```python
from build123d import *

# Parameters (mm, degrees)
F0_W     = 110
F0_H     = 2
F1_DEPTH = 412
F2_W     = 455.0662100537
F2_H     = 4
F3_DEPTH = 16


with BuildPart() as f1:
    # F0 (on Top) → F1 (new body)
    with BuildSketch(Plane.XY):
        with Locations((-49.3745803833, 21.5659940839)):
            Rectangle(F0_W, F0_H)
        Polygon((5.6254196167, 22.5659940839), (5.6254196167, 20.5659940839), (465.6254196127, 100.5659940832), (453.9570552758, 100.5659940832), align=None)
    extrude(amount=F1_DEPTH)

    # F2 (on face) → F3 (join)
    with BuildSketch(Plane(origin=(-3.6453815607, 20.9530753552, 0), x_dir=(-0.9852008911, -0.1714036294, 0), z_dir=(-0.1714036294, 0.9852008911, 0))):
        with Locations((-236.9431667321, 410)):
            Rectangle(F2_W, F2_H)
    extrude(amount=F3_DEPTH)


solid = f1.part
```
Geometry check sheet. Reference: the model listing, model coordinates, mm. A direction names the side the tool comes from. Round coordinates to 2 decimals unless told otherwise and drop trailing zeros. Loops run counter-clockwise (first coordinate to the right, second up) from the corner with the lowest first, then second, coordinate; pieces in that order, holes last. Notation, with made-up numbers: (61.5, 47) - (112.5, 47) arc R9 cw to (112.5, 55) - close; hole circle Ø1 at (16, 6.5). An arc over 180 degrees is marked (long way). Write each question's results on one line, items separated by ' | '. Start each with the question number.
Q1. Gauge pin test, flat ends, axial feed: P1, Ø9.5, axis at x = 457.5, z = 128.5, coming from the +Y side; P2, Ø5, axis at x = 267, z = 229.5, coming from the +Y side; P3, Ø10, axis at x = 342.5, z = 261, coming from the -Y side. Record the tip position at first contact, or that the pin passes through.
Q2. Thickness scan on line 1 (Z direction, x = 53, y = 43); line 2 (Y direction, x = -66.5, z = 181); line 3 (Y direction, x = 182.5, z = 23.5). Record the ranges inside material, lowest first. Write a range as [from, to].
Q3. Cross-section at B-B on x = 13.5. Enter the section's corners in (y, z).
Q4. Access from +Z, -Z, +X, -X, +Y, -Y to the whole of each face (thin tool, end or side, straight path). Record for faces 1 (the flat face through (-50, 20.566, 203)), 2 (the flat face through (232, 70, 408)).
Q5. Cross-section at A-A on z = 117. Enter the section's corners in (x, y).
Answers below:
1) P1: stops at y = 100.57 | P2: stops at y = 68.47 | P3: stops at y = 78.28
2) line 1: z = [408, 412] | line 2: y = [20.57, 22.57] | line 3: y = [51.33, 53.34]
3) outline: (21.94, 0) - (23.94, 0) - (23.94, 408) - (40.18, 408) - (40.18, 412) - (21.94, 412) - close
4) face 1: +Z, -Z, +X, -X, -Y | face 2: -Z, -X, +Y
5) outline: (-104.37, 20.57) - (5.63, 20.57) - (465.63, 100.57) - (453.96, 100.57) - (5.63, 22.57) - (-104.37, 22.57) - close
